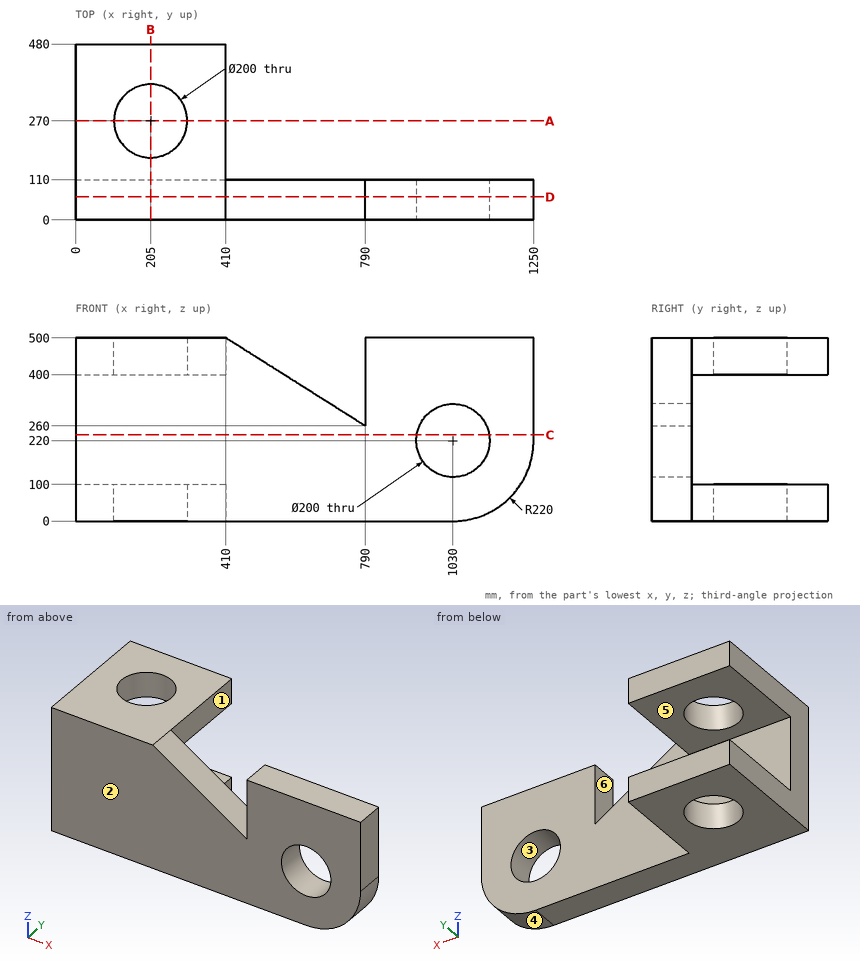
Geometry check sheet. Reference: drawing and pictorial views, mm from the part's lowest x, y, z. A direction names the side the tool comes from. Coordinates: 2 decimals unless noted, no trailing zeros. Order: outer loops, then holes, each group sorted by start corner. A loop starts at its lowest first (then second) coordinate and runs counter-clockwise, first axis right, second up. Notation, with made-up numbers: (50, -19) -> (109, -19) arc R21 cw to (109, 20) -> close; hole circle Ø8 at (-1, 46.25). An arc over 180 degrees is marked (long way). Write item = value, one per line. Start each with the question number.
1) Cross-section at D-D (y = 63). Enter the section's corners in (x, z), then the cut area to 3 significant figures.
2) Go/stop test with a flat-tipped pin: P1, Ø6, axis at x = 259, z = 332, coming from the +Y side. Record where the tip stops, or that it passes through.
3) Cross-section at B-B (x = 205). Enter the section's corners in (y, z), then the cut area to 3 significant figures.
4) Access from +Z, -Z, +X, -X, +Y, -Y to the whole of each face (thin tool, end or side, straight path). Record for the marked faces 4, 5 and 6.
5) Cross-section at A-A (y = 270). Enter the section's corners in (x, z), then the cut area to 3 significant figures.
6) Material ranges on L1, parallel to X at y = 269, z = 95 (3 decimals); L2, parallel to Z at x = 1030, y = 62.5; L3, parallel to Y at x = 205, z = 428, recorded low to high.
7) Cross-section at C-C (z = 235.5). Enter the section's corners in (x, y), then the cut area to 3 significant figures.
8) Mould release check, pull along X, two halves, no side actions. Record for the marked faces 1, 2 and 3: +X half, -X half, draft (parallel to the pull), parting line (faces both ways), or undercut.
Ans:
q1.outline = (0, 0) -> (1030, 0) arc R220 ccw to (1250, 220) -> (1250, 500) -> (790, 500) -> (790, 260) -> (410, 500) -> (0, 500) -> close; hole circle Ø200 at (1030, 220)
q1.area = 538,000 mm²
q2.P1 = 110
q3.outline = (0, 0) -> (170, 0) -> (170, 100) -> (110, 100) -> (110, 400) -> (170, 400) -> (170, 500) -> (0, 500) -> close; (370, 0) -> (480, 0) -> (480, 100) -> (370, 100) -> close; (370, 400) -> (480, 400) -> (480, 500) -> (370, 500) -> close
q3.area = 89,000 mm²
q4.face_4 = -Z, +X, +Y, -Y
q4.face_5 = +X, -X, +Y
q4.face_6 = +Z, +Y, -Y
q5.outline = (0, 0) -> (105, 0) -> (105, 100) -> (0, 100) -> close; (0, 400) -> (105, 400) -> (105, 500) -> (0, 500) -> close; (305, 0) -> (410, 0) -> (410, 100) -> (305, 100) -> close; (305, 400) -> (410, 400) -> (410, 500) -> (305, 500) -> close
q5.area = 42,000 mm²
q6.L1 = 0 to 105.005, 304.995 to 410
q6.L2 = 0 to 120, 320 to 500
q6.L3 = 0 to 170, 370 to 480
q7.outline = (0, 0) -> (931.21, 0) -> (931.21, 110) -> (0, 110) -> close; (1128.79, 0) -> (1250, 0) -> (1250, 110) -> (1128.79, 110) -> close
q7.area = 116,000 mm²
q8.face_1 = +X half
q8.face_2 = draft
q8.face_3 = undercut
